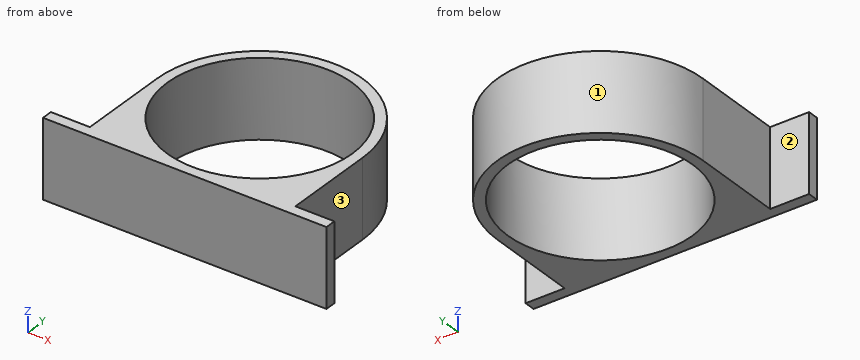
```python
from build123d import *

# Parameters (mm, degrees)
SKETCH1_R           = 33.375
SKETCH1_R_2         = 30.007470458
BOSS_EXTRUDE1_DEPTH = 25.3
BASE_W              = 92.07
BASE_H              = 3.511684016
BOSS_EXTRUDE3_DEPTH = 25.3
SKETCH7_W           = 66.75
SKETCH7_H           = 25.3
BOSS_EXTRUDE4_DEPTH = 33.3
SKETCH2_R           = 30
CUT_EXTRUDE4_DEPTH  = 33.3


with BuildPart() as part:
    # Sketch1 → Boss-Extrude1 (new body)
    with BuildSketch(Plane.XY):
        Circle(SKETCH1_R)
        Circle(SKETCH1_R_2, mode=Mode.SUBTRACT)
        Circle(SKETCH1_R_2)
    extrude(amount=BOSS_EXTRUDE1_DEPTH)

    # Base → Boss-Extrude3 (add)
    with BuildSketch(Plane.XY):
        with Locations((0, -31.619157992)):
            Rectangle(BASE_W, BASE_H)
    extrude(amount=BOSS_EXTRUDE3_DEPTH)

    # Sketch7 → Boss-Extrude4 (add)
    with BuildSketch(Plane(origin=(0, 0, 0), x_dir=(1, 0, 0), z_dir=(0, 1, 0))):
        with Locations((0, -12.65)):
            Rectangle(SKETCH7_W, SKETCH7_H)
    extrude(amount=-BOSS_EXTRUDE4_DEPTH)

    # Sketch2 → Cut-Extrude4 (cut)
    with BuildSketch(Plane(origin=(0, 0, 0), x_dir=(-1, 0, 0), z_dir=(0, 0, -1))):
        Circle(SKETCH2_R)
    extrude(amount=-CUT_EXTRUDE4_DEPTH, mode=Mode.SUBTRACT)


solid = part.part
```
Input: part model. Units: mm. Frame: model coordinates. Face numbers are marked on the shaded views. A direction names the side the tool comes from. Give positions to 0.01 mm unless a question says otherwise; leave off trailing zeros. Order: outer loops, then holes, each group sorted by start corner. A loop starts at its lowest first (then second) coordinate and runs counter-clockwise, first axis right, second up. Notation, with made-up numbers: M -32,51 L -14,51 A9 ccw -14,59 Z; hole C -21.5,3 d1. An arc over 180 degrees is marked long. Return JSON: item names as keys, results as strings.
Item 1: Cut plane A-A (x = 0). Return loops of the section in (y, z) (3 decimals).
Solutions:
{"outline": "M -33.375,0 L -30,0 L -30,25.3 L -33.375,25.3 Z; M 30,0 L 33.375,0 L 33.375,25.3 L 30,25.3 Z"}
Item 2: Cut plane C-C (y = 10). Return loops of the section in (x, z), then the cut area to 3 significant figures.
Solutions:
{"outline": "M -31.84,0 L -28.28,0 L -28.28,25.3 L -31.84,25.3 Z; M 28.28,0 L 31.84,0 L 31.84,25.3 L 28.28,25.3 Z", "area": "180 mm^2"}
Item 3: First-contact query: P1, Ø5, axis at y = -13, z = 11, coming from the -X side (3 decimals); P2, Ø10, axis at x = 34, z = 18, coming from the +Y side; P3, Ø8, axis at y = 2, z = 5, coming from the +X side (3 decimals). Flat tips, straight axial feed; report the tip coordinate or a pass-through.
Solutions:
{"P1": "x = -33.375", "P2": "y = 16.52", "P3": "x = 33.375"}
Item 4: Access query for the marked faces 1, 2 and 3. Directions: +Z, -Z, +X, -X, +Y, -Y. A direction counts if a zero-diameter tool reaches every point of the face in a straight line with its end or side. Return the directions, or none.
Solutions:
{"face 1": "+Z, -Z, +Y", "face 2": "+Z, -Z, -X, +Y", "face 3": "+Z, -Z, +X, +Y"}
Item 5: Ray query, probe 1 along Y at (x, z) = (0, 12.5) (3 decimals); probe 2 along X at (y, z) = (24, 16.75); probe 3 along X at (y, z) = (-13, 24) (3 decimals). Return the intervals inside material, ascending.
Solutions:
{"probe 1": "-33.375 to -30, 30 to 33.375", "probe 2": "-23.19 to -18, 18 to 23.19", "probe 3": "-33.375 to -27.037, 27.037 to 33.375"}
Item 6: Cut plane B-B (z = 1.75). Return loops of the section in (x, y) (3 decimals), then the cut area to 3 significant figures.
Solutions:
{"outline": "M -46.035,-33.375 L 46.035,-33.375 L 46.035,-29.863 L 33.375,-29.863 L 33.375,0 A33.375 ccw -33.375,0 L -33.375,-29.863 L -46.035,-29.863 Z; hole C 0,0 d60", "area": "1,240 mm^2"}
